Part model, mm, in its own coordinate system. A direction names the side the tool comes from. Round coordinates to 2 decimals unless told otherwise and drop trailing zeros. Loops run counter-clockwise (first coordinate to the right, second up) from the corner with the lowest first, then second, coordinate; pieces in that order, holes last.
from build123d import *

# Parameters (mm, degrees)
F0_W     = 72.9848642368
F0_H     = 75.440466404
F1_DEPTH = 76.2
F3_D     = 25.4
F4_W     = 25.4
F4_H     = 25.4
F5_DEPTH = 12.7
F7_R     = 12.7
F8_DEPTH = 12.7


# Not quite as in the source:
# - a length typed as a fraction of an inch, garbled in the dataset ("3 / 203.2 mm" for 3/8 in), is restored


with BuildPart() as f1:
    # F0 (on Front) → F1 (new body)
    with BuildSketch(Plane.XZ):
        with Locations((39.7899424424, 37.720233202)):
            Rectangle(F0_W, F0_H)
    extrude(amount=F1_DEPTH)

    # F3 (through all)
    with Locations(Plane.XY.offset(75.440466404)):
        with Locations((36.5493223071, -37.9619333167)):
            Hole(F3_D / 2)

    # F4 (on face) → F5 (join)
    with BuildSketch(Plane.XZ.offset(76.2)):
        with Locations((40.9810889382, 43.4622988105)):
            Rectangle(F4_W, F4_H)
    extrude(amount=F5_DEPTH)

    # F7 (on face) → F8 (join)
    with BuildSketch(Plane.YZ.offset(76.2823745608)):
        with Locations((-36.2048484385, 37.505440414)):
            Circle(F7_R)
    extrude(amount=F8_DEPTH)


solid = f1.part
1) Mould opens along Y. For faces 1 (the face through (45.91, -29.38, 37.19)), 2 (the face through (39, 0, 38)), 3 (the face through (28.281, -82, 43)) say: released by +Y, released by -Y, zero draft, split by the parting line, or undercut.
Values:
face 1: undercut
face 2: released by +Y
face 3: zero draft
2) Tool access for faces 4 (the face through (53.681, -82, 43)), 5 (the face through (82.54, -30.34, 26.24)), 6 (the face through (41, -82, 30.762)), 7 (the face through (41, -82, 56.162)): list every direction of +Z, -Z, +X, -X, +Y, -Y with a clear straight run to the whole face (end or side of a thin tool).
Values:
face 4: +Z, -Z, +X, -Y
face 5: +X
face 6: -Z, +X, -X, -Y
face 7: +Z, +X, -X, -Y
3) Slice it at A-A, the plane x = 42.5. Give the cut face in (y, z), then the cut area to 3 significant figures.
Values:
outline: (-88.9, 30.76) - (-76.2, 30.76) - (-76.2, 0) - (-49.18, 0) - (-49.18, 75.44) - (-76.2, 75.44) - (-76.2, 56.16) - (-88.9, 56.16) - close; (-26.74, 0) - (0, 0) - (0, 75.44) - (-26.74, 75.44) - close
area: 4,380 mm2
4) Slice it at D-D, the plane z = 40. Give the cut face in (x, y), then the cut area to 3 significant figures.
Values:
outline: (3.3, -76.2) - (28.28, -76.2) - (28.28, -88.9) - (53.68, -88.9) - (53.68, -76.2) - (76.28, -76.2) - (76.28, -48.66) - (88.98, -48.66) - (88.98, -23.75) - (76.28, -23.75) - (76.28, 0) - (3.3, 0) - close; hole circle Ø25.4 at (36.55, -37.96)
area: 5,690 mm2
5) Slice it at B-B, the plane y = -36. Give the cut face in (x, z), then the cut area to 3 significant figures.
Values:
outline: (3.3, 0) - (24, 0) - (24, 75.44) - (3.3, 75.44) - close; (49.1, 0) - (76.28, 0) - (76.28, 24.81) - (88.98, 24.81) - (88.98, 50.2) - (76.28, 50.2) - (76.28, 75.44) - (49.1, 75.44) - close
area: 3,940 mm2
6) Slice it at C-C, the plane z = 28. Give the cut face in (x, y), then the cut area to 3 significant figures.
Values:
outline: (3.3, -76.2) - (76.28, -76.2) - (76.28, -44.63) - (88.98, -44.63) - (88.98, -27.78) - (76.28, -27.78) - (76.28, 0) - (3.3, 0) - close; hole circle Ø25.4 at (36.55, -37.96)
area: 5,270 mm2
7) Drop flat-ended pins along their axis: pin 1 Ø8 at (x, y) = (36, -30) entering from -Z; pin 2 Ø6.5 at (y, z) = (-80, 40) entering from -X; pin 3 Ø10 at (x, y) = (43.5, -84.5) entering from +Z; pin 4 Ø8 at (y, z) = (-22.5, 12.5) entering from +X. Give the stop position or say it passes through.
Values:
pin 1: passes through
pin 2: stops at x = 28.28
pin 3: stops at z = 56.16
pin 4: stops at x = 76.28
8) Wall check: line 1 along Y through (x, z) = (36.5, 43.5); line 2 along X through (y, z) = (-52, 4.5); line 3 along Y through (x, z) = (21, 16). Give the ranges that are in metal, low to high.
Values:
line 1: y = -88.9 to -50.66, -25.26 to 0
line 2: x = 3.3 to 76.28
line 3: y = -76.2 to 0
